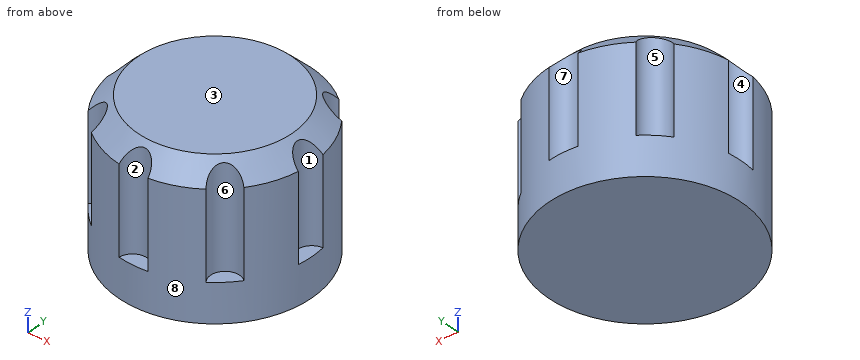
from build123d import *

# Parameters (mm, degrees)
CYLINDER001_R     = 1.5
CYLINDER001_DEPTH = 20
ARRAY_COUNT       = 8
CYLINDER_R        = 10
CYLINDER_DEPTH    = 15
CHAMFER_SIZE      = 2


with BuildPart() as array:
    # Cylinder001 → Cylinder001 (new body)
    with BuildSketch(Plane(origin=(10, 0, 0), x_dir=(1, 0, 0), z_dir=(0, 0, 1))):
        Circle(CYLINDER001_R)
    extrude(amount=CYLINDER001_DEPTH)

    # Array: Array ×8 about axis
    array_axis = Axis((0, 0, 0), (0, 0, 1))


with BuildPart() as array_1:
    add(array.part)
    for i in range(1, ARRAY_COUNT):
        add(array.part.rotate(array_axis, i * 360 / ARRAY_COUNT))


with BuildPart() as array_2:
    # Array placement: moved
    add(array_1.part.moved(Location((0, 0, 4))))


with BuildPart() as cut:
    # Cylinder → Cylinder (new body)
    with BuildSketch(Plane.XY):
        Circle(CYLINDER_R)
    extrude(amount=CYLINDER_DEPTH)

    # Chamfer
    chamfer_edges = [cut.edges().sort_by_distance(p)[0] for p in [
        (-10, 0, 15),
    ]]
    chamfer(chamfer_edges, length=CHAMFER_SIZE)

    # Cut: cut Array
    add(array_2.part, mode=Mode.SUBTRACT)


solid = cut.part
Verification items for the finished model (mm, model axes). Face numbers are marked on the shaded views. A direction names the side the tool comes from. Coordinates: 2 decimals unless noted, no trailing zeros. Order: outer loops, then holes, each group sorted by start corner. A loop starts at its lowest first (then second) coordinate and runs counter-clockwise, first axis right, second up. Notation, with made-up numbers: (-29, -22) -> (1, -22) arc R6 cw to (1, -12) -> close; hole circle Ø10 at (61, -15.5). An arc over 180 degrees is marked (long way). Put each result on its own line as item: value. Start each with the question number.
1. Material ranges on L1, parallel to X at y = 0, z = 13.75; L2, parallel to X at y = -0.25, z = 3.25; L3, parallel to Z at x = -7.5, y = 6.5, recorded low to high. Write a range as [from, to].
2. Mould release check, pull along Y, two halves, no side actions. Record for the marked faces 6, 7 and 8: released by +Y, released by -Y, zero draft, split by the parting line, or undercut.
3. Access from +Z, -Z, +X, -X, +Y, -Y to the whole of each face (thin tool, end or side, straight path). Record for the marked faces 1, 2, 3, 4 and 5.
4. Go/stop test with flat-tipped pins: pin 1 Ø1.5 at (y, z) = (4, 8.5) entering from +X; pin 2 Ø2.5 at (x, y) = (7, -7) entering from +Z; pin 3 Ø3 at (y, z) = (-5.5, 12) entering from -X. Record where each tip stops, or that it passes through.
5. Cross-section at A-A, the plane x = 0. Record the boundary of the cut face in (y, z).
6. Cross-section at C-C, the plane z = 2.5. Record the boundary of the cut face in (x, y), then the cut area to 3 significant figures.
Computed:
1. L1: [-8.5, 8.5]
1. L2: [-10, 10]
1. L3: [0, 4]
2. face 6: undercut
2. face 7: released by +Y
2. face 8: split by the parting line
3. face 1: +Z, +X
3. face 2: +Z, -Y
3. face 3: +Z, +X, -X, +Y, -Y
3. face 4: +Z, -X
3. face 5: +Z
4. pin 1: x = 9.46
4. pin 2: z = 4
4. pin 3: x = -9.17
5. outline: (-10, 0) -> (10, 0) -> (10, 4) -> (8.5, 4) -> (8.5, 14.5) -> (8, 15) -> (-8, 15) -> (-8.5, 14.5) -> (-8.5, 4) -> (-10, 4) -> close
6. outline: circle Ø20 at (0, 0)
6. area: 314 mm2
